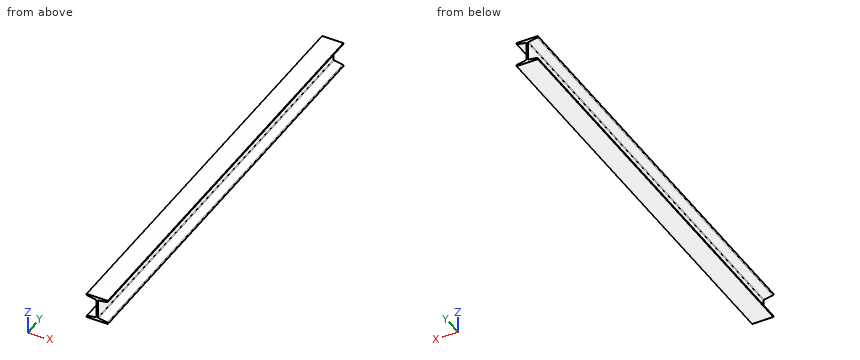
from build123d import *

# Parameters (mm, degrees)
EXTRUDE_DEPTH = 1280
FILLET_R      = 2


with BuildPart() as part:
    # Sketch → Extrude (new body)
    with BuildSketch(Plane.XZ):
        Polygon((-31.75, 38.1), (31.75, 38.1), (31.75, 33.3375), (2.38125, 28.575), (2.38125, -28.575), (31.75, -33.3375), (31.75, -38.1), (-31.75, -38.1), (-31.75, -33.3375), (-2.38125, -28.575), (-2.38125, 28.575), (-31.75, 33.3375), align=None)
    extrude(amount=-EXTRUDE_DEPTH)

    # Fillet
    fillet_edges = [part.edges().sort_by_distance(p)[0] for p in [
        (31.75, 640, 33.3375),
        (2.38125, 640, 28.575),
        (2.38125, 640, -28.575),
        (31.75, 640, -33.3375),
        (-31.75, 640, -33.3375),
        (-2.38125, 640, -28.575),
        (-2.38125, 640, 28.575),
        (-31.75, 640, 33.3375),
    ]]
    fillet(fillet_edges, radius=FILLET_R)


solid = part.part
Verification items for the finished model (mm, model axes). Give positions to 0.01 mm unless a question says otherwise; leave off trailing zeros. Write each loop counter-clockwise with the first axis right and the second up, starting at its lowest first coordinate (ties: lowest second). Pieces come first, ordered by that corner, then holes. Notation, with made-up numbers: M 42,79.25 L 79,79.25 A9 ccw 79,95.25 Z; hole C 53,48.5 d7. An arc over 180 degrees is marked long. Write item = value, one per line.
(1) Material ranges on line 1 (Z direction, x = 13, y = 55.5); line 2 (Z direction, x = -11, y = 75); line 3 (X direction, y = 259, z = -14), recorded low to high.
Found:
line_1 = -38.1 to -30.3, 30.3 to 38.1
line_2 = -38.1 to -29.97, 29.97 to 38.1
line_3 = -2.38 to 2.38
(2) Sectioned sample at A-A (x = -19.5). Record the cut outline in (y, z), then the cut area to 3 significant figures.
Found:
outline = M 0,-38.1 L 1280,-38.1 L 1280,-31.35 L 0,-31.35 Z; M 0,31.35 L 1280,31.35 L 1280,38.1 L 0,38.1 Z
area = 17,300 mm2
(3) Go/stop test with a flat-tipped pin: pin 1 Ø16 at (y, z) = (860, 9.5) entering from -X. Record where the tip stops, or that it passes through.
Found:
pin_1 = -2.38
(4) Sectioned sample at C-C (z = -4.5). Record the cut outline in (x, y).
Found:
outline = M -2.38,0 L 2.38,0 L 2.38,1280 L -2.38,1280 Z
(5) Sectioned sample at B-B (y = 511). Record the cut outline in (x, z).
Found:
outline = M -31.75,-38.1 L 31.75,-38.1 L 31.75,-35.04 A2 ccw 30.07,-33.07 L 4.06,-28.85 A2 cw 2.38,-26.87 L 2.38,26.87 A2 cw 4.06,28.85 L 30.07,33.07 A2 ccw 31.75,35.04 L 31.75,38.1 L -31.75,38.1 L -31.75,35.04 A2 ccw -30.07,33.07 L -4.06,28.85 A2 cw -2.38,26.87 L -2.38,-26.87 A2 cw -4.06,-28.85 L -30.07,-33.07 A2 ccw -31.75,-35.04 Z
